```python
from build123d import *

# Parameters (mm, degrees)
SKETCH1_W                = 25.5
SKETCH1_H                = 43
BOSS_EXTRUDE1_DEPTH      = 1.6
BOSS_EXTRUDE2_DEPTH      = 8.6
BOSS_EXTRUDE2_DEPTH_BACK = 3.1
SKETCH2_W                = 2.5
SKETCH2_H                = 20
SKETCH3_W                = 3
SKETCH3_H                = 3
BOSS_EXTRUDE3_DEPTH      = 1
FILLET1_R                = 1.5
CHAMFER1_SIZE            = 2.5


with BuildPart() as part:
    # Sketch1 → Boss-Extrude1 (new body)
    with BuildSketch(Plane(origin=(0, 0, 0), x_dir=(1, 0, 0), z_dir=(0, 1, 0))):
        with Locations((12.75, 21.5)):
            Rectangle(SKETCH1_W, SKETCH1_H)
    extrude(amount=BOSS_EXTRUDE1_DEPTH)

    # Sketch2 → Boss-Extrude2 (add, two sides: drawn at the far end of the back side and taken through both)
    with BuildSketch(Plane.XZ.offset(-BOSS_EXTRUDE2_DEPTH_BACK)):
        with Locations((1.25, -12.7)):
            Rectangle(SKETCH2_W, SKETCH2_H)
        with Locations((24.25, -12.7)):
            Rectangle(SKETCH2_W, SKETCH2_H)
    extrude(amount=BOSS_EXTRUDE2_DEPTH + BOSS_EXTRUDE2_DEPTH_BACK)

    # Sketch3 → Boss-Extrude3 (add)
    with BuildSketch(Plane(origin=(0, 1.6, 0), x_dir=(1, 0, 0), z_dir=(0, 1, 0))):
        with Locations((12.75, 38.8)):
            Rectangle(SKETCH3_W, SKETCH3_H)
    extrude(amount=BOSS_EXTRUDE3_DEPTH)

    # Fillet1
    fillet1_edges = [part.edges().sort_by_distance(p)[0] for p in [
        (0, 0.8, -43),
        (25.5, 0.8, -43),
    ]]
    fillet(fillet1_edges, radius=FILLET1_R)

    # Chamfer1
    chamfer1_edges = [part.edges().sort_by_distance(p)[0] for p in [
        (25.5, 0.8, 0),
    ]]
    chamfer(chamfer1_edges, length=CHAMFER1_SIZE)


solid = part.part
```
Geometry check sheet. Reference: the model listing, model coordinates, mm. A direction names the side the tool comes from. Give positions to 0.01 mm unless a question says otherwise; leave off trailing zeros. Write each loop counter-clockwise with the first axis right and the second up, starting at its lowest first coordinate (ties: lowest second). Pieces come first, ordered by that corner, then holes. Notation, with made-up numbers: (3.25, 49) -> (38.25, 49) arc R26 cw to (38.25, 81) -> close; hole circle Ø2 at (16, 78). An arc over 180 degrees is marked (long way). Use one line per item in the form item = value.
Item 1: Sectioned sample at D-D on x = 18. Enter the section's corners in (y, z).
Results list:
outline = (0, -43) -> (1.6, -43) -> (1.6, 0) -> (0, 0) -> close
Item 2: Mould release check, pull along X, two halves, no side actions. Record for faces 5 (the flat face through (24, -4, -2.7)), 6 (the cylindrical face through (0.43, 0.81, -42.55)), 7 (the flat face through (13, 0, -22)), 8 (the flat face through (13, 1.6, -22)): released by +X, released by -X, zero draft, split by the parting line, or undercut.
Results list:
face_5 = zero draft
face_6 = released by -X
face_7 = undercut
face_8 = undercut
Item 3: Sectioned sample at C-C on z = -9. Enter the section's corners in (x, y), plus the area to 3 significant figures.
Results list:
outline = (0, -8.6) -> (2.5, -8.6) -> (2.5, 0) -> (23, 0) -> (23, -8.6) -> (25.5, -8.6) -> (25.5, 3.1) -> (23, 3.1) -> (23, 1.6) -> (2.5, 1.6) -> (2.5, 3.1) -> (0, 3.1) -> close
area = 91.3 mm2
Item 4: Sectioned sample at A-A on y = -6. Enter the section's corners in (x, z).
Results list:
outline = (0, -22.7) -> (2.5, -22.7) -> (2.5, -2.7) -> (0, -2.7) -> close; (23, -22.7) -> (25.5, -22.7) -> (25.5, -2.7) -> (23, -2.7) -> close
Item 5: Sectioned sample at B-B on x = 12.5. Enter the section's corners in (y, z), plus the area to 3 significant figures.
Results list:
outline = (0, -43) -> (1.6, -43) -> (1.6, -40.3) -> (2.6, -40.3) -> (2.6, -37.3) -> (1.6, -37.3) -> (1.6, 0) -> (0, 0) -> close
area = 71.8 mm2
Item 6: Access from +Z, -Z, +X, -X, +Y, -Y to the whole of each face (thin tool, end or side, straight path). Record for faces 1 (the flat face through (24, 2, -2.7)), 2 (the flat face through (13, 2, -40.3)), 3 (the flat face through (24, -4, -22.7)), 4 (the flat face through (2.5, 2, -13)).
Results list:
face_1 = +Z, +X, -X, +Y
face_2 = -Z, +X, -X, +Y
face_3 = -Z, +X, -X, -Y
face_4 = +Z, -Z, +Y
Item 7: Scan lines: line 1 (X direction, y = -1, z = -15.5); line 2 (Y direction, x = 19, z = -39); line 3 (X direction, y = 1.75, z = -40). Record each from-to range of solid material in increasing order.
Results list:
line_1 = 0 to 2.5, 23 to 25.5
line_2 = 0 to 1.6
line_3 = 11.25 to 14.25
Item 8: Depth check by flat-ended pin: pin 1 Ø0.5 at (y, z) = (2, -38.5) entering from -X; pin 2 Ø2 at (x, y) = (18.5, -1.5) entering from -Z; pin 3 Ø0.8 at (x, y) = (1.5, 2.5) entering from +Z; pin 4 Ø3 at (x, y) = (1, -6) entering from -Z. Enter the tip coordinate at first touch or a pass-through.
Results list:
pin_1 = 11.25
pin_2 = through
pin_3 = -2.7
pin_4 = -22.7
